Could you check a few things on this model? Use its own coordinates, in mm. Face numbers are marked on the shaded views. Give positions to 0.01 mm unless a question says otherwise; leave off trailing zeros. Order: outer loops, then holes, each group sorted by start corner. A loop starts at its lowest first (then second) coordinate and runs counter-clockwise, first axis right, second up. Notation, with made-up numbers: M -33,-16 L 15,-16 A25 cw 15,10 Z; hole C 79.25,33 d8. An arc over 180 degrees is marked long. Use a Markdown table: item, result. Add a question column.
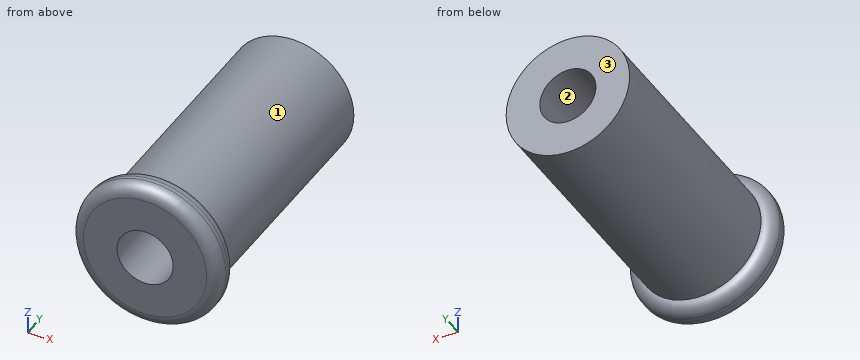
```python
from build123d import *

# Parameters (mm, degrees)
F0_R        = 2.0088927205
F0_R_2      = 0.9130728347
F1_DEPTH    = 8.89
F0_R_3      = 2.413
F2_DEPTH    = 0.94454
F3_S5_R     = 2.0088927205
F3_T6_DEPTH = 5


# Not quite as in the source:
# - a fillet or chamfer that OpenCascade refuses, or shapes differently, is made with other operations: its cross-section is extruded or revolved along the edge and cut away or added


with BuildPart() as f1:
    # F0 (on Front) → F1 (new body)
    with BuildSketch(Plane.XZ):
        Circle(F0_R)
        Circle(F0_R_2, mode=Mode.SUBTRACT)
    extrude(amount=-F1_DEPTH)

    # F0 (on Front) → F2 (join)
    with BuildSketch(Plane.XZ):
        Circle(F0_R_3)
        Circle(F0_R, mode=Mode.SUBTRACT)
    extrude(amount=-F2_DEPTH)

    # F3: fillet of radius 0.4064 on 2 edges, made by hand


with BuildPart() as f3_tool2:
    # F3_s3 → F3_t4 (revolve)
    with BuildSketch(Plane.XY):
        with BuildLine():
            ThreePointArc((2.0066, 0.94454), (2.2939681959, 0.8255081959), (2.413, 0.53814))
            Line((2.413, 0.53814), (2.413, 0.94454))
            Line((2.413, 0.94454), (2.0066, 0.94454))
        make_face()
    revolve(axis=Axis((0, 0.94454, 0), (0, -1, 0)))

    # F3_s5 → F3_t6 (cut, symmetric)
    with BuildSketch(Plane.XZ.offset(-0.6)):
        Circle(F3_S5_R)
    extrude(amount=F3_T6_DEPTH, both=True, mode=Mode.SUBTRACT)


with BuildPart() as f1_1:
    add(f1.part)

    # F3_t1: cut F3_tool2
    add(f3_tool2.part, mode=Mode.SUBTRACT)

    # F3_s7 → F3_t8 (revolve, cut)
    with BuildSketch(Plane.XY):
        with BuildLine():
            ThreePointArc((2.413, 0.4064), (2.2939681959, 0.1190318041), (2.0066, 0))
            Line((2.0066, 0), (2.413, 0))
            Line((2.413, 0), (2.413, 0.4064))
        make_face()
    revolve(axis=Axis((0, 0, 0), (0, -1, 0)), mode=Mode.SUBTRACT)


solid = f1_1.part
```
1) Suppose I cut it at C-C on y = 3. Please give me the cut outline in (x, z), and give its area (3 significant figures).
2) Suppose I cut it at A-A on x = 0. Please give me the cut outline in (y, z).
3) Suppose I cut it at B-B on z = 0. Please give me the cut outline in (x, y).
4) For pin 1 (1 mm diameter, centred on x = -1.5, y = 2.5, fed in from +Z); pin 2 (1 mm diameter, centred on x = -2, y = 7, fed in from +Z), each with a flat end and sliding along its axis, tell me the tip position at first contact or that it passes through.
5) Please list where these lines run through material, in increasing order: line 1 (Z direction, x = 0, y = 6.25); line 2 (X direction, y = 1.25, z = -0.5); line 3 (Y direction, x = -1.6, z = -1.6). Write a range as from..to.
6) We'd pull the mould along X, two halves only. Please class the marked faces 1, 2 and 3: pulls with the +X half, pulls with the -X half, needs draft (parallel to the pull), parting line crosses it, or undercut.
Values found:
| question | item | result |
|---|---|---|
| 1 | outline | C 0,0 d4.02; hole C 0,0 d1.83 |
| 1 | area | 10.1 mm^2 |
| 2 | outline | M 0,-2.01 A0.41 ccw 0.41,-2.41 L 0.54,-2.41 A0.41 ccw 0.94,-2.01 L 8.89,-2.01 L 8.89,-0.91 L 0,-0.91 Z; M 0,0.91 L 8.89,0.91 L 8.89,2.01 L 0.94,2.01 A0.41 ccw 0.54,2.41 L 0.41,2.41 A0.41 ccw 0,2.01 Z |
| 3 | outline | M -2.41,0.41 A0.41 ccw -2.01,0 L -0.91,0 L -0.91,8.89 L -2.01,8.89 L -2.01,0.94 A0.41 ccw -2.41,0.54 Z; M 0.91,0 L 2.01,0 A0.41 ccw 2.41,0.41 L 2.41,0.54 A0.41 ccw 2.01,0.94 L 2.01,8.89 L 0.91,8.89 Z |
| 4 | pin 1 | stops at z = 1.74 |
| 4 | pin 2 | stops at z = 1.34 |
| 5 | line 1 | z = -2.01..-0.91, 0.91..2.01 |
| 5 | line 2 | x = -1.95..-0.76, 0.76..1.95 |
| 5 | line 3 | y = 0.09..0.85 |
| 6 | face 1 | parting line crosses it |
| 6 | face 2 | undercut |
| 6 | face 3 | needs draft |
